```python
from build123d import *

# Parameters (mm, degrees)
ESBO_O1_R                  = 1.5
RESSALTO_EXTRUS_O1_DEPTH   = 14
FILETE4_R                  = 5
FILETE5_R                  = 2
ESBO_O5_R                  = 4
RESSALTO_EXTRUS_O4_DEPTH   = 4
ESBO_O6_R                  = 1
CORTE_EXTRUS_O3_DEPTH      = 5
CORTE_EXTRUS_O3_DEPTH_BACK = 32
CORTE_EXTRUS_O4_DEPTH      = 1
CORTE_EXTRUS_O5_DEPTH      = 1


with BuildPart() as part:
    # Esboço1 → Ressalto-extrusão1 (new body)
    with BuildSketch(Plane(origin=(0, 0, 0), x_dir=(1, 0, 0), z_dir=(0, 1, 0))):
        Polygon((15.5, 15.5), (-8.5, 15.5), (-8.5, 8.5), (-15.5, 8.5), (-15.5, -15.5), (15.5, -15.5), align=None)
        with Locations((-10, -10)):
            Circle(ESBO_O1_R, mode=Mode.SUBTRACT)
        with Locations((10, -10)):
            Circle(ESBO_O1_R, mode=Mode.SUBTRACT)
    extrude(amount=RESSALTO_EXTRUS_O1_DEPTH)

    # Filete4
    filete4_edges = [part.edges().sort_by_distance(p)[0] for p in [
        (15.5, 7, 15.5),
        (-15.5, 7, 15.5),
    ]]
    fillet(filete4_edges, radius=FILETE4_R)

    # Filete5
    filete5_edges = [part.edges().sort_by_distance(p)[0] for p in [
        (-15.5, 7, -8.5),
    ]]
    fillet(filete5_edges, radius=FILETE5_R)

    # Esboço5 → Ressalto-extrusão4 (add)
    with BuildSketch(Plane(origin=(15.5, 0, 0), x_dir=(0, 0, -1), z_dir=(1, 0, 0))):
        with Locations((11.49, 7)):
            Circle(ESBO_O5_R)
    extrude(amount=RESSALTO_EXTRUS_O4_DEPTH)

    # Esboço6 → Corte-extrusão3 (cut, two sides)
    with BuildSketch(Plane(origin=(15.5, 0, 0), x_dir=(0, 0, -1), z_dir=(1, 0, 0))) as corte_extrus_o3_sk:
        with Locations((11.49, 7)):
            Circle(ESBO_O6_R)
    extrude(amount=CORTE_EXTRUS_O3_DEPTH, mode=Mode.SUBTRACT)
    extrude(corte_extrus_o3_sk.sketch, amount=-CORTE_EXTRUS_O3_DEPTH_BACK, mode=Mode.SUBTRACT)

    # Esboço7 → Corte-extrusão4 (cut)
    with BuildSketch(Plane(origin=(0, 14, 0), x_dir=(1, 0, 0), z_dir=(0, 1, 0))):
        Polygon((-5, 1), (-5, -1), (1, -1), (1, -2), (5, 0), (1, 2), (1, 1), align=None)
    extrude(amount=-CORTE_EXTRUS_O4_DEPTH, mode=Mode.SUBTRACT)

    # Esboço9 → Corte-extrusão5 (cut)
    with BuildSketch(Plane.XZ):
        Polygon((-5.123658733, -0.978330013), (0.876341267, -0.978330013), (0.876341267, -1.978330013), (4.876341267, 0.021669987), (0.876341267, 2.021669987), (0.876341267, 1.021669987), (-5.123658733, 1.021669987), align=None)
    extrude(amount=-CORTE_EXTRUS_O5_DEPTH, mode=Mode.SUBTRACT)


solid = part.part
```
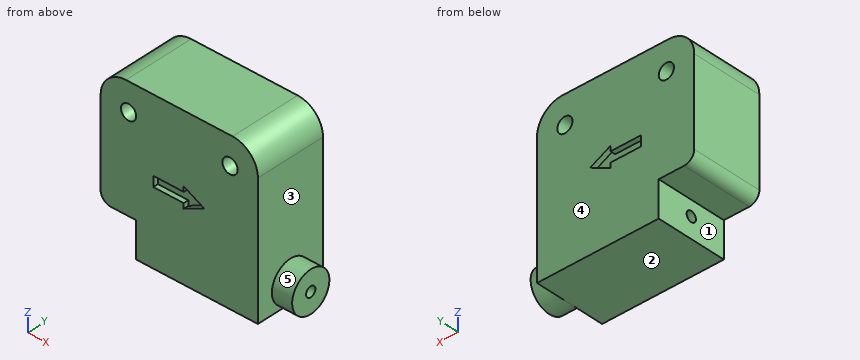
Geometry: final body of the model. Coordinates: model frame, mm. Face numbers are marked on the shaded views. A direction names the side the tool comes from. Coordinates: 2 decimals unless noted, no trailing zeros. Order: outer loops, then holes, each group sorted by start corner. A loop starts at its lowest first (then second) coordinate and runs counter-clockwise, first axis right, second up. Notation, with made-up numbers: (65.5, -29.75) - (117.5, -29.75) arc R33 ccw to (117.5, 9.25) - close; hole circle Ø4 at (54, 67.5). An arc over 180 degrees is marked (long way). Write each question's results on one line, items separated by ' | '.
1) Pull-direction query (Y, two-part tool) for the marked faces 3, 4 and 5; classes: pulls with the +Y half, pulls with the -Y half, needs draft (parallel to the pull), parting line crosses it, or undercut.
Results list:
face 3: needs draft | face 4: pulls with the +Y half | face 5: parting line crosses it
2) Section B-B, the plane x = -10. Return loops of the section in (y, z).
Results list:
outline: (0, -8.5) - (14, -8.5) - (14, 8.5) - (0, 8.5) - close; (0, 11.5) - (14, 11.5) - (14, 15.5) - (0, 15.5) - close
3) Set-up query: the marked faces 1 and 2. Return all of +Z, -Z, +X, -X, +Y, -Y with unobstructed straight access to the full face (end or side cutting, diameter ignored); none if empty.
Results list:
face 1: -Z, -X, +Y, -Y | face 2: -Z, +X, -X, +Y, -Y
4) Section A-A, the plane x = 10. Return loops of the section in (y, z).
Results list:
outline: (0, -15.5) - (14, -15.5) - (14, 8.5) - (0, 8.5) - close; (0, 11.5) - (14, 11.5) - (14, 15.5) - (0, 15.5) - close; hole circle Ø2 at (7, -11.49)
5) Section D-D, the plane z = -11.49. Return loops of the section in (x, y).
Results list:
outline: (-8.5, 0) - (15.5, 0) - (15.5, 3) - (19.5, 3) - (19.5, 6) - (-8.5, 6) - close; (-8.5, 8) - (19.5, 8) - (19.5, 11) - (15.5, 11) - (15.5, 14) - (-8.5, 14) - close
6) Section C-C, the plane y = 7. State how many separate pieces and enclosed holes the cut face has, plus the area to 3 significant figures.
Results list:
separate pieces: 2 | enclosed holes: 2 | area: 862 mm^2
7) Pin query (flat end, axial travel): pin 1 (0.5 mm diameter, centred on y = 13.5, z = 0, fed in from +X); pin 2 (4 mm diameter, centred on x = -11, y = 3.5, fed in from -Z); pin 3 (2.5 mm diameter, centred on y = 7, z = -11.49, fed in from -X). Return the tip coordinate at first contact, or that it passes through.
Results list:
pin 1: x = 15.5 | pin 2: z = -8.5 | pin 3: x = -8.5
8) Line query: line 1 (X direction, y = 7, z = 10); line 2 (Z direction, x = -10, y = 5.5); line 3 (X direction, y = 6, z = 9.5). Output: solid intervals per line, ascending. Write a range as from..to.
Results list:
line 1: -15.5..-11.5, -8.5..8.5, 11.5..15.5 | line 2: -8.5..8.5, 11.5..15.5 | line 3: -15.5..-11.41, -8.59..8.59, 11.41..15.5
